Can you work these out from the drawing? Everything is in mm from the part's minimum corner. Round coordinates to 2 decimals unless told otherwise and drop trailing zeros. Order: outer loops, then holes, each group sorted by start corner. A loop starts at its lowest first (then second) coordinate and runs counter-clockwise, first axis right, second up. Notation, with made-up numbers: (-10.5, 68.25) -> (10.5, 68.25) arc R4 ccw to (10.5, 72.25) -> close; hole circle Ø11 at (-25, 60). An arc over 180 degrees is marked (long way). One line per item, written item: value.
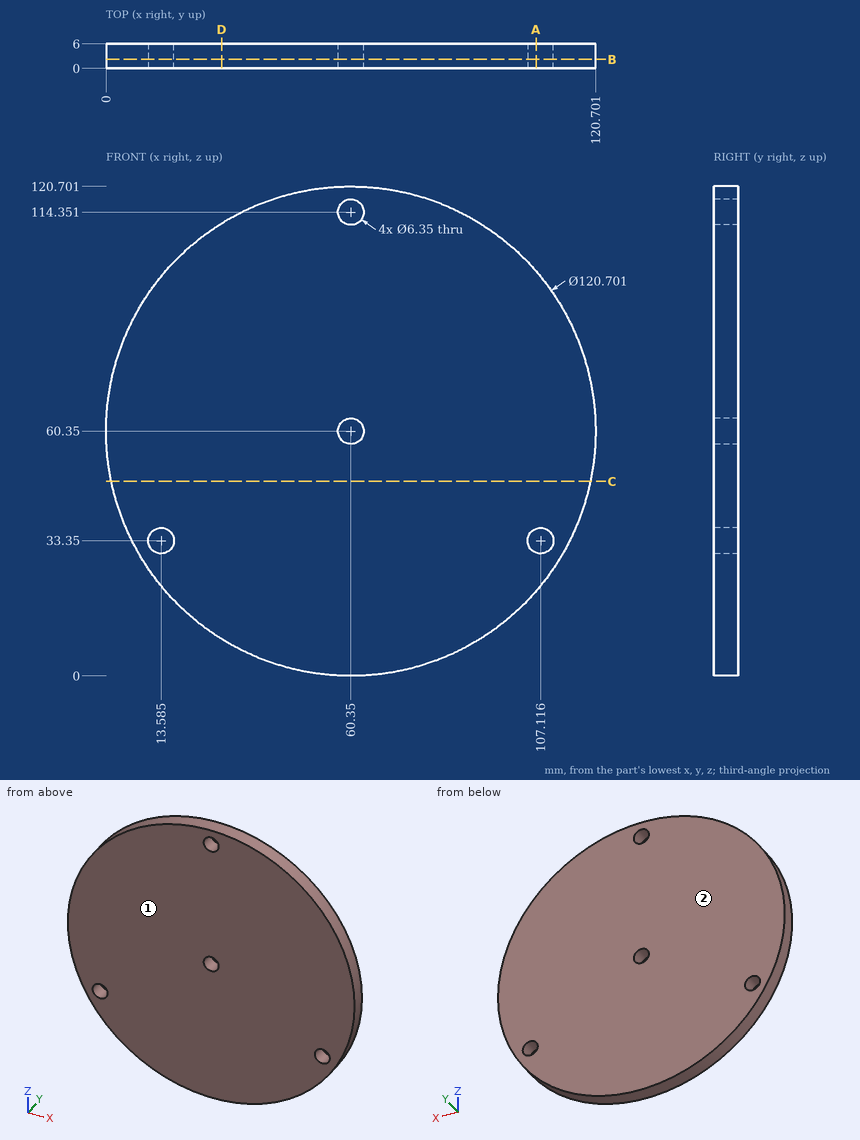
Q1. I want a section at C-C on z = 48. List the corners of the cut face in (x, y) for me.
Answers below:
outline: (1.28, 0) -> (119.42, 0) -> (119.42, 6) -> (1.28, 6) -> close
Q2. We'd pull the mould along Y, two halves only. Please class the marked faces 1 and 2: released by +Y, released by -Y, zero draft, split by the parting line, or undercut.
Answers below:
face 1: released by -Y
face 2: released by +Y
Q3. I want a section at D-D on x = 28.5. List the corners of the cut face in (y, z) for me.
Answers below:
outline: (0, 9.09) -> (6, 9.09) -> (6, 111.61) -> (0, 111.61) -> close
Q4. Will these pins go through, and if not, where does the flat tip stop? pin 1 Ø10 at (x, z) = (60.35, 114.35) entering from -Y; pin 2 Ø1.5 at (x, y) = (26.5, 4) entering from +Z; pin 3 Ø3 at (y, z) = (1, 64.5) entering from +X; pin 4 Ø3 at (y, z) = (2, 74) entering from +X (1 decimal).
Answers below:
pin 1: y = 0
pin 2: z = 110.81
pin 3: x = 120.64
pin 4: x = 119.5
Q5. I want a section at A-A on x = 106. List the corners of the cut face in (y, z) for me (1 decimal), plus the area to 3 significant figures.
Answers below:
outline: (0, 20.9) -> (6, 20.9) -> (6, 30.4) -> (0, 30.4) -> close; (0, 36.3) -> (6, 36.3) -> (6, 99.8) -> (0, 99.8) -> close
area: 438 mm^2
Q6. I want a section at B-B on y = 2.2. Give the number of separate pieces and of enclosed holes in the cut face, plus the area to 3 significant figures.
Answers below:
separate pieces: 1
enclosed holes: 4
area: 11,300 mm^2
Q7. Please list where these lines run through material, in increasing order: line 1 along X through (y, z) = (1.9, 61); line 2 along Z through (x, y) = (11, 0.3) (1 decimal); line 3 along Z through (x, y) = (71.5, 3.35).
Answers below:
line 1: 0 to 57.24, 63.46 to 120.7
line 2: 25.6 to 31.5, 35.2 to 95.1
line 3: 1.04 to 119.66
